Could you check a few things on this model? Use its own coordinates, in mm. Face numbers are marked on the shaded views. A direction names the side the tool comes from. Give positions to 0.01 mm unless a question says otherwise; leave off trailing zeros. Order: outer loops, then holes, each group sorted by start corner. A loop starts at its lowest first (then second) coordinate and runs counter-clockwise, first axis right, second up. Notation, with made-up numbers: (-27.75, 63.25) -> (13.25, 63.25) arc R25 cw to (13.25, 81.25) -> close; hole circle Ø4 at (1.25, -30.5). An arc over 180 degrees is marked (long way). One line per item, written item: value.
```python
from build123d import *

# Parameters (mm, degrees)
F1_DEPTH = 5


# Not quite as in the source:
# - ends of sketch curves that miss each other by under 0.0002 mm in the source are joined


with BuildPart() as f1:
    # F0 (on Top) → F1 (new body)
    with BuildSketch(Plane.XY):
        with BuildLine():
            ThreePointArc((1.8058852177, 17.4790926703), (1.8279530148, 4.8720604744), (-7.149820085, -3.9787777878))
            ThreePointArc((-7.149820085, -3.9787777878), (-8.2306223723, -4.5782907715), (-9.1313488192, -5.4246011501))
            Line((-9.1313488192, -5.4246011501), (-12.197101, -9.119353))
            Line((-12.197101, -9.119353), (-12.197101, -15.150279))
            Line((-12.197101, -15.150279), (-3.447101, -15.150279))
            Line((-3.447101, -15.150279), (-3.447101, -27.150279))
            Line((-3.447101, -27.150279), (6.552899, -27.150279))
            Line((6.552899, -27.150279), (6.552899, -15.150279))
            Line((6.552899, -15.150279), (12.197102, -5.240307))
            Line((12.197102, -5.240307), (12.197102, 27.150279))
            Line((12.197102, 27.150279), (3.197102, 27.150279))
            Line((3.197102, 27.150279), (1.562377, 20.643277))
            ThreePointArc((1.562377, 20.643277), (1.4264287194, 19.0413526341), (1.8058852177, 17.4790926703))
        make_face()
    extrude(amount=F1_DEPTH)


solid = f1.part
```
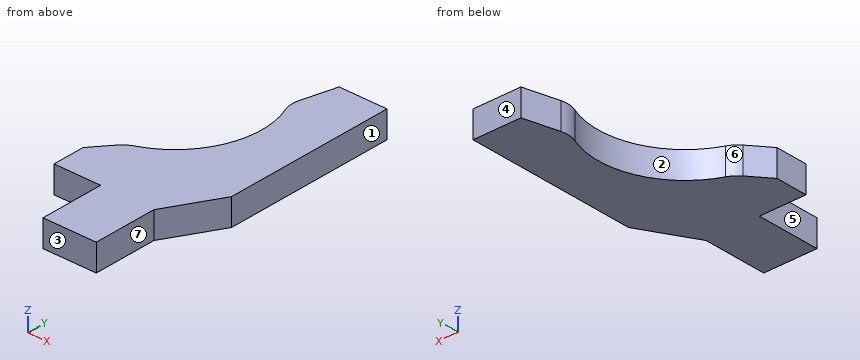
1) We'd pull the mould along Y, two halves only. Please class the marked faces 1, 2, 3 and 4: +Y half, -Y half, draft (parallel to the pull), parting line (faces both ways), or undercut.
Answer below:
face 1: draft
face 2: undercut
face 3: -Y half
face 4: +Y half
2) Suppose I cut it at B-B, the plane y = -21.5. Write out the boundary of the cut face in (x, z), then the cut area to 3 significant figures.
Answer below:
outline: (-3.45, 0) -> (6.55, 0) -> (6.55, 5) -> (-3.45, 5) -> close
area: 50.0 mm2
3) For the marked faces 5, 6 and 7, which set-ups out of +Z, -Z, +X, -X, +Y, -Y let a thin tool reach every point of the face, with its end or its side?
Answer below:
face 5: +Z, -Z, -X, -Y
face 6: +Z, -Z, -X, +Y
face 7: +Z, -Z, +X, -Y
4) For P1, Ø1.5, axis at x = -6, z = 2.5, coming from the -Y side; P2, Ø1.5, axis at y = -20, z = 3.5, coming from the +X side, each with a flat end and sliding along its axis, tell me the tip position at first contact or that it passes through.
Answer below:
P1: stops at y = -15.15
P2: stops at x = 6.55
5) Suppose I cut it at A-A, the plane z = 3.1. Write out the boundary of the cut face in (x, y) (3 decimals).
Answer below:
outline: (-12.197, -15.15) -> (-3.447, -15.15) -> (-3.447, -27.15) -> (6.553, -27.15) -> (6.553, -15.15) -> (12.197, -5.24) -> (12.197, 27.15) -> (3.197, 27.15) -> (1.562, 20.643) arc R5 ccw to (1.806, 17.479) arc R16.298 cw to (-7.15, -3.979) arc R5 ccw to (-9.131, -5.425) -> (-12.197, -9.119) -> close
6) If I drill on line 1 along X through (y, z) = (-24.5, 1.65); line 2 along X through (y, z) = (11, 3.7); line 3 along Y through (x, z) = (1.25, 1.35), over which ranges is the centre line in solid material (lowest first)?
Answer below:
line 1: x = -3.45 to 6.55
line 2: x = 3.08 to 12.2
line 3: y = -27.15 to 3.64
7) Suppose I cut it at C-C, the plane x = -4. Write out the boundary of the cut face in (y, z), then the cut area to 3 significant figures.
Answer below:
outline: (-15.15, 0) -> (-2.29, 0) -> (-2.29, 5) -> (-15.15, 5) -> close
area: 64.3 mm2
